The listing builds one solid part. Answer for the finished solid, in the listing's coordinates (mm). A direction names the side the tool comes from. Give positions to 0.01 mm unless a question says otherwise; leave off trailing zeros. Order: outer loops, then holes, each group sorted by start corner. A loop starts at its lowest first (then second) coordinate and runs counter-clockwise, first axis right, second up. Notation, with made-up numbers: (25.5, -6) - (48.5, -6) arc R32 cw to (48.5, 25) - close; hole circle Ø9 at (-17, 66.5). An arc over 180 degrees is marked (long way). Use a Markdown table: item, result. Add a question column.
1) Flat-ended cylindrical pins translate along their axes: pin 1 (1.5 mm diameter, centred on x = 35.5, z = 92.5, fed in from -Y); pin 2 (2 mm diameter, centred on x = 74.5, z = 91.5, fed in from -Y); pin 3 (1.5 mm diameter, centred on x = 51.5, z = 62.5, fed in from +Y). Find the tip coordinate at first contact, or state that the pin passes through.
2) Straight lines are drawn through the part: line 1 (Y direction, x = 11, z = 61.5); line 2 (Z direction, x = 25, y = 7.5); line 3 (Z direction, x = 24, y = 3.75). For each, find the intervals that lie inside material, in ascending order.
3) For faces 1 (the face through (23.528, 7.93, 185.326)), 2 (the face through (65, 13, 10)), determine the directions among +Z, -Z, +X, -X, +Y, -Y from which every point of the face is accessible in a straight line to the end or side of a thin tool.
4) Find section B-B, the plane y = 4.75. Determine the outline of the cut face in (x, z).
5) Find section D-D, the plane z = 110.5. Determine the outline of the cut face in (x, y), plus the area to 4 significant figures.
6) Find section A-A, the plane z = 10. Determine the outline of the cut face in (x, y).
7) Find section C-C, the plane x = 65. Determine the outline of the cut face in (y, z), plus the area to 3 significant figures.
from build123d import *

# Parameters (mm, degrees)
SKETCH1_W           = 75
SKETCH1_H           = 3
BOSS_EXTRUDE1_DEPTH = 200
SKETCH2_R           = 4.9
BOSS_EXTRUDE2_DEPTH = 10
SKETCH5_W           = 2.5
SKETCH5_H           = 200
CUT_EXTRUDE2_DEPTH  = 1


with BuildPart() as part:
    # Sketch1 → Boss-Extrude1 (new body)
    with BuildSketch(Plane.XY):
        with Locations((37.5, 1.5)):
            Rectangle(SKETCH1_W, SKETCH1_H)
    extrude(amount=BOSS_EXTRUDE1_DEPTH)

    # Sketch2 → Boss-Extrude2 (add)
    with BuildSketch(Plane(origin=(0, 3, 0), x_dir=(1, 0, 0), z_dir=(0, 1, 0))):
        with Locations(Location((25, -190, 0), (0, 0, 90))):
            Circle(SKETCH2_R)
        with Locations(Location((65, -10, 0), (0, 0, 90))):
            Circle(SKETCH2_R)
        with Locations((165, -190)):
            Circle(SKETCH2_R)
        with Locations((85, -190)):
            Circle(SKETCH2_R)
        with Locations((-27.5, -10)):
            Circle(SKETCH2_R)
    extrude(amount=BOSS_EXTRUDE2_DEPTH)


with BuildPart() as boss_extrude2_kept_piece:
    # of the separate pieces the step leaves, the one the design keeps (boss_extrude2_pieces_kept)
    add(part.part.solids().sort_by_distance((0, 0, 0))[0])

    # Sketch5 → Cut-Extrude2 (cut)
    with BuildSketch(Plane.XZ):
        with Locations((73.75, 100)):
            Rectangle(SKETCH5_W, SKETCH5_H)
    extrude(amount=-CUT_EXTRUDE2_DEPTH, mode=Mode.SUBTRACT)


solid = boss_extrude2_kept_piece.part
The answers:
| question | item | result |
|---|---|---|
| 1 | pin 1 | y = 0 |
| 1 | pin 2 | y = 1 |
| 1 | pin 3 | y = 3 |
| 2 | line 1 | 0 to 3 |
| 2 | line 2 | 185.1 to 194.9 |
| 2 | line 3 | 185.2 to 194.8 |
| 3 | face 1 | +Y |
| 3 | face 2 | +Z, -Z, +X, -X, +Y |
| 4 | outline | circle Ø9.8 at (25, 190); circle Ø9.8 at (65, 10) |
| 5 | outline | (0, 0) - (72.5, 0) - (72.5, 1) - (75, 1) - (75, 3) - (0, 3) - close |
| 5 | area | 222.5 mm2 |
| 6 | outline | (0, 0) - (72.5, 0) - (72.5, 1) - (75, 1) - (75, 3) - (69.9, 3) - (69.9, 13) - (60.1, 13) - (60.1, 3) - (0, 3) - close |
| 7 | outline | (0, 0) - (3, 0) - (3, 5.1) - (13, 5.1) - (13, 14.9) - (3, 14.9) - (3, 200) - (0, 200) - close |
| 7 | area | 698 mm2 |
